```python
from build123d import *

# Parameters (mm, degrees)
SKETCH1_W                                        = 25.65
SKETCH1_H                                        = 14
SKETCH1_W_2                                      = 14
SKETCH1_H_2                                      = 34.73
BOSS_EXTRUDE1_DEPTH                              = 42.65
SKETCH2_R                                        = 6.425
CUT_EXTRUDE1_DEPTH                               = 42.65
SKETCH3_W                                        = 1.9
SKETCH3_H                                        = 30
CUT_EXTRUDE2_DEPTH                               = 42.65
SKETCH4_R                                        = 6.425
CUT_EXTRUDE3_DEPTH                               = 42.65
SKETCH5_W                                        = 32
SKETCH5_H                                        = 1.9
CUT_EXTRUDE4_DEPTH                               = 42.65
M3_CLEARANCE_HOLE1_D                             = 3.6
M3_CLEARANCE_HOLE1_DEPTH                         = 10
M3_CLEARANCE_HOLE1_CSINK_D                       = 3.65
M3_CLEARANCE_HOLE1_CSINK_ANGLE                   = 90
M3_CLEARANCE_HOLE1_TIP                           = 1.081549114
SKETCH9_W                                        = 61.993652624
SKETCH9_H                                        = 40.55348858
CUT_EXTRUDE5_DEPTH                               = 61.688696641
SKETCH10_R                                       = 1.825
BOSS_EXTRUDE2_DEPTH                              = 10
CBORE_FOR_1_4_SOCKET_HEAD_CAP_SCREW1_D           = 6.7564
CBORE_FOR_1_4_SOCKET_HEAD_CAP_SCREW1_CBORE_D     = 11.1125
CBORE_FOR_1_4_SOCKET_HEAD_CAP_SCREW1_CBORE_DEPTH = 6.35
SKETCH14_R                                       = 5
CUT_EXTRUDE6_DEPTH                               = 5
CHAMFER1_SIZE                                    = 2


with BuildPart() as part:
    # Sketch1 → Boss-Extrude1 (new body)
    with BuildSketch(Plane.XY):
        with Locations((-12.825, -7)):
            Rectangle(SKETCH1_W, SKETCH1_H)
        with Locations((7, -17.365)):
            Rectangle(SKETCH1_W_2, SKETCH1_H_2)
    extrude(amount=BOSS_EXTRUDE1_DEPTH)

    # Sketch2 → Cut-Extrude1 (cut)
    with BuildSketch(Plane.XZ.offset(14)):
        with Locations((-14.665, 27.725)):
            Circle(SKETCH2_R)
    extrude(amount=-CUT_EXTRUDE1_DEPTH, mode=Mode.SUBTRACT)

    # Sketch3 → Cut-Extrude2 (cut)
    with BuildSketch(Plane.XZ.offset(14)):
        with Locations((-16.7, 27.65)):
            Rectangle(SKETCH3_W, SKETCH3_H)
    extrude(amount=-CUT_EXTRUDE2_DEPTH, mode=Mode.SUBTRACT)

    # Sketch4 → Cut-Extrude3 (cut)
    with BuildSketch(Plane.ZY):
        with Locations(Location((18.725, -21.745, 0), (0, 0, 270))):
            Circle(SKETCH4_R)
    extrude(amount=-CUT_EXTRUDE3_DEPTH, mode=Mode.SUBTRACT)

    # Sketch5 → Cut-Extrude4 (cut)
    with BuildSketch(Plane.ZY):
        with Locations((26.65, -25.78)):
            Rectangle(SKETCH5_W, SKETCH5_H)
    extrude(amount=-CUT_EXTRUDE4_DEPTH, mode=Mode.SUBTRACT)

    # M3 Clearance Hole1
    with Locations(Plane(origin=(0, 0, 0), x_dir=(-1, 0, 0), z_dir=(0, 0, -1))):
        with Locations((1.1, -5.25), (13.5, -5.25), (-6.99, -21.8)):
            CounterSinkHole(M3_CLEARANCE_HOLE1_D / 2, M3_CLEARANCE_HOLE1_CSINK_D / 2, depth=M3_CLEARANCE_HOLE1_DEPTH, counter_sink_angle=M3_CLEARANCE_HOLE1_CSINK_ANGLE)
            with Locations((0, 0, -(M3_CLEARANCE_HOLE1_DEPTH + M3_CLEARANCE_HOLE1_TIP / 2))):  # 118° drill point
                Cone(0, M3_CLEARANCE_HOLE1_D / 2, M3_CLEARANCE_HOLE1_TIP, mode=Mode.SUBTRACT)

    # Sketch9 → Cut-Extrude5 (cut, through all)
    with BuildSketch(Plane(origin=(0, 0, 0), x_dir=(1, 0, 0), z_dir=(0, 1, 0))):
        with Locations((-5.42180131, -25.55674429)):
            Rectangle(SKETCH9_W, SKETCH9_H)
    extrude(amount=-CUT_EXTRUDE5_DEPTH, mode=Mode.SUBTRACT)

    # Sketch10 → Boss-Extrude2 (add)
    with BuildSketch(Plane(origin=(0, 0, 0), x_dir=(-1, 0, 0), z_dir=(0, 0, -1))):
        Polygon((25.65, 0), (-14, 0), (-14, -34.73), (0, -34.73), (0, -14), (25.65, -14), align=None)
        with Locations((1.1, -5.25)):
            Circle(SKETCH10_R, mode=Mode.SUBTRACT)
        with Locations((13.5, -5.25)):
            Circle(SKETCH10_R, mode=Mode.SUBTRACT)
        with Locations((-6.99, -21.8)):
            Circle(SKETCH10_R, mode=Mode.SUBTRACT)
    extrude(amount=BOSS_EXTRUDE2_DEPTH)

    # CBORE for 1_4 Socket Head Cap Screw1 (through all)
    with Locations(Plane.XY.offset(5.28)):
        with Locations((6.597752863, -9.469911877)):
            CounterBoreHole(CBORE_FOR_1_4_SOCKET_HEAD_CAP_SCREW1_D / 2, CBORE_FOR_1_4_SOCKET_HEAD_CAP_SCREW1_CBORE_D / 2, CBORE_FOR_1_4_SOCKET_HEAD_CAP_SCREW1_CBORE_DEPTH)

    # Sketch14 → Cut-Extrude6 (cut)
    with BuildSketch(Plane(origin=(0, 0, -10), x_dir=(-1, 0, 0), z_dir=(0, 0, -1))):
        with Locations((1.1, -5.25)):
            Circle(SKETCH14_R)
        with Locations((13.5, -5.25)):
            Circle(SKETCH14_R)
        with Locations((-6.99, -21.8)):
            Circle(SKETCH14_R)
    extrude(amount=-CUT_EXTRUDE6_DEPTH, mode=Mode.SUBTRACT)

    # Chamfer1
    chamfer1_edges = [part.edges().sort_by_distance(p)[0] for p in [
        (9.975952863, -9.469911877, -1.07),
    ]]
    chamfer(chamfer1_edges, length=CHAMFER1_SIZE)


solid = part.part
```
Model file for the job. Use its own axes, mm. A direction names the side the tool comes from. Give positions to 0.01 mm unless a question says otherwise; leave off trailing zeros. Loops run counter-clockwise (first coordinate to the right, second up) from the corner with the lowest first, then second, coordinate; pieces in that order, holes last. Notation, with made-up numbers: M 56.5,11.25 L 71.5,11.25 A16 cw 71.5,20.25 Z; hole C 74.25,-23 d2. An arc over 180 degrees is marked long. Use one line per item in the form item = value.
Item 1: Slice it at B-B on x = -13.5. List the corners of the cut face in (y, z) (3 decimals), and give its area (3 significant figures).
Filled in:
outline = M -14,-10 L -10.25,-10 L -10.25,-5 L -7.075,-5 L -7.075,0 L -7.05,0.025 L -7.05,5.28 L -14,5.28 Z; M -3.45,0.025 L -3.425,0 L -3.425,-5 L -0.25,-5 L -0.25,-10 L 0,-10 L 0,5.28 L -3.45,5.28 Z
area = 127 mm^2
Item 2: Flat gauge pins, fed straight in: pin 1 Ø6 at (x, y) = (-1.1, -5.25) entering from +Z; pin 2 Ø4.5 at (x, y) = (-13.5, -5.25) entering from -Z; pin 3 Ø8 at (x, y) = (-9, -20.5) entering from +Z; pin 4 Ø9 at (x, y) = (6.5, -8.5) entering from +Z. Where does each tip first touch, or does it go through?
Filled in:
pin_1 = 5.28
pin_2 = -5
pin_3 = through
pin_4 = -1.07
Item 3: Two-plate mould, pull along X, no slides. Class faces 1 (the cylindrical face through (2.87, -8.29, -7.54)), 2 (the flat face through (-1, -13, -10)), 3 (the flat face through (-25.65, -7, -2)), 4 (the flat face through (14, -17, -2)): released by +X, released by -X, zero draft, split by the parting line, or undercut.
Filled in:
face_1 = undercut
face_2 = zero draft
face_3 = released by -X
face_4 = released by +X
Item 4: Slice it at D-D on x = 6.5. Give the number of separate pieces and of enclosed holes in the cut face, and give its area (3 significant figures).
Filled in:
separate_pieces = 3
enclosed_holes = 0
area = 310 mm^2
Item 5: Slice it at A-A on y = -21.8. List the corners of the cut face in (x, z) (3 decimals).
Filled in:
outline = M 0,-10 L 1.99,-10 L 1.99,-5 L 5.165,-5 L 5.165,0 L 5.19,0.025 L 5.19,5.28 L 0,5.28 Z; M 8.79,0.025 L 8.815,0 L 8.815,-5 L 11.99,-5 L 11.99,-10 L 14,-10 L 14,5.28 L 8.79,5.28 Z
Item 6: Drill centre lines: L1, parallel to Y at x = -1.1, z = -7.5; L2, parallel to X at y = -21.8, z = 2.1; L3, parallel to X at y = -27.5, z = 2.5. Where is each one in solid material? Low to high.
Filled in:
L1 = -14 to -10.25, -0.25 to 0
L2 = 0 to 5.19, 8.79 to 14
L3 = 0 to 14
Item 7: Which spindle directions (+Z, -Z, +X, -X, +Y, -Y) get a long thin tool onto all of the face, cutting with end or side? Do faces 5 (the flat face through (7, -24, -5)), 6 (the flat face through (-6, 0, -2)), 7 (the flat face through (0, -25, -2)). Say none if no direction does.
Filled in:
face_5 = -Z
face_6 = +Z, -Z, +X, -X, +Y
face_7 = +Z, -Z, -X, -Y
Item 8: Slice it at C-C on z = 4.25. List the corners of the cut face in (x, y), and give its area (3 significant figures).
Filled in:
outline = M -25.65,-14 L 0,-14 L 0,-34.73 L 14,-34.73 L 14,0 L -25.65,0 Z; hole C -13.5,-5.25 d3.6; hole C -1.1,-5.25 d3.6; hole C 6.6,-9.47 d11.11; hole C 6.99,-21.8 d3.6
area = 718 mm^2
